from build123d import *

# Parameters (mm, degrees)
SKETCH1_R           = 31.5
BOSS_EXTRUDE1_DEPTH = 55
CUT_EXTRUDE1_START  = 53
SKETCH1_4_R         = 31.5
SKETCH1_4_R_2       = 9
CUT_EXTRUDE1_DEPTH  = 2
SKETCH1_5_R         = 4
BOSS_EXTRUDE2_DEPTH = 29.525
SKETCH1_7_R         = 2
CUT_EXTRUDE2_DEPTH  = 10
CUT_EXTRUDE3_START  = 53
SKETCH1_10_R        = 1.5
CUT_EXTRUDE3_DEPTH  = 5
CHAMFER1_SIZE       = 5
CHAMFER1_SIZE2      = 12
CHAMFER2_SIZE       = 7
CHAMFER2_SIZE2      = 16
BOSS_EXTRUDE4_START = 75
SKETCH1_11_R        = 4
BOSS_EXTRUDE4_DEPTH = 20


with BuildPart() as part:
    # Sketch1 → Boss-Extrude1 (new body)
    with BuildSketch(Plane(origin=(0, 0, 0), x_dir=(1, 0, 0), z_dir=(0, 1, 0))):
        with Locations(Location((0, 0, 0), (0, 0, 270))):
            Circle(SKETCH1_R)
    extrude(amount=BOSS_EXTRUDE1_DEPTH)

    # Sketch1<4> → Cut-Extrude1 (cut)
    with BuildSketch(Plane(origin=(0, 0, 0), x_dir=(1, 0, 0), z_dir=(0, 1, 0)).offset(CUT_EXTRUDE1_START)):
        with Locations(Location((0, 0, 0), (0, 0, 270))):
            Circle(SKETCH1_4_R)
        with Locations(Location((0, 0, 0), (0, 0, 270))):
            Circle(SKETCH1_4_R_2, mode=Mode.SUBTRACT)
    extrude(amount=CUT_EXTRUDE1_DEPTH, mode=Mode.SUBTRACT)

    # Sketch1<5> → Boss-Extrude2 (add)
    with BuildSketch(Plane(origin=(0, 0, 0), x_dir=(1, 0, 0), z_dir=(0, 1, 0))):
        with Locations(Location((0, 0, 0), (0, 0, 270))):
            Circle(SKETCH1_5_R)
    extrude(amount=-BOSS_EXTRUDE2_DEPTH)

    # Sketch1<7> → Cut-Extrude2 (cut)
    with BuildSketch(Plane(origin=(0, 0, 0), x_dir=(1, 0, 0), z_dir=(0, 1, 0))):
        with Locations(Location((22.2, 0, 0), (0, 0, 270))):
            Circle(SKETCH1_7_R)
        with Locations(Location((0, 22.2, 0), (0, 0, 270))):
            Circle(SKETCH1_7_R)
        with Locations(Location((-22.2, 0, 0), (0, 0, 270))):
            Circle(SKETCH1_7_R)
        with Locations(Location((0, -22.2, 0), (0, 0, 270))):
            Circle(SKETCH1_7_R)
    extrude(amount=CUT_EXTRUDE2_DEPTH, mode=Mode.SUBTRACT)

    # Sketch1<10> → Cut-Extrude3 (cut)
    with BuildSketch(Plane(origin=(0, 0, 0), x_dir=(1, 0, 0), z_dir=(0, 1, 0)).offset(CUT_EXTRUDE3_START)):
        with Locations(Location((-11.7, 0, 0), (0, 0, 270))):
            Circle(SKETCH1_10_R)
        with Locations(Location((0, 11.7, 0), (0, 0, 270))):
            Circle(SKETCH1_10_R)
        with BuildLine():
            ThreePointArc((13.2, 0), (11.7, 1.5), (10.2, 0))
            Line((10.2, 0), (13.2, 0))
        make_face()
        with BuildLine():
            Line((13.2, 0), (10.2, 0))
            ThreePointArc((10.2, 0), (11.7, -1.5), (13.2, 0))
        make_face()
        with Locations(Location((0, -11.7, 0), (0, 0, 270))):
            Circle(SKETCH1_10_R)
    extrude(amount=-CUT_EXTRUDE3_DEPTH, mode=Mode.SUBTRACT)

    # Chamfer1
    chamfer1_edges = [part.edges().sort_by_distance(p)[0] for p in [
        (0, 0, -31.5),
    ]]
    chamfer1_side = [part.faces().sort_by_distance(p)[0] for p in [
        (0, 0, -30.609045456),
    ]]
    chamfer(chamfer1_edges, length=CHAMFER1_SIZE, length2=CHAMFER1_SIZE2, reference=chamfer1_side[0])

    # Chamfer2
    chamfer2_edges = [part.edges().sort_by_distance(p)[0] for p in [
        (0, 53, -31.5),
    ]]
    chamfer2_side = [part.faces().sort_by_distance(p)[0] for p in [
        (0, 32.5, -31.5),
    ]]
    chamfer(chamfer2_edges, length=CHAMFER2_SIZE, length2=CHAMFER2_SIZE2, reference=chamfer2_side[0])

    # Sketch1<11> → Boss-Extrude4 (add)
    with BuildSketch(Plane(origin=(0, 0, 0), x_dir=(1, 0, 0), z_dir=(0, 1, 0)).offset(BOSS_EXTRUDE4_START)):
        with Locations(Location((0, 0, 0), (0, 0, 270))):
            Circle(SKETCH1_11_R)
    extrude(amount=-BOSS_EXTRUDE4_DEPTH)


solid = part.part
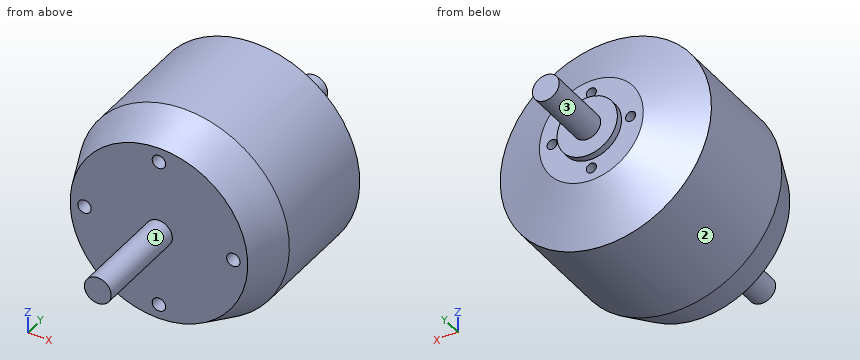
The listing builds one solid part. Answer for the finished solid, in the listing's coordinates (mm). Face numbers are marked on the shaded views. A direction names the side the tool comes from. Round coordinates to 2 decimals unless told otherwise and drop trailing zeros. Write each loop counter-clockwise with the first axis right and the second up, starting at its lowest first coordinate (ties: lowest second). Pieces come first, ordered by that corner, then holes. Notation, with made-up numbers: M 15,36.25 L 56,36.25 A32 cw 56,62.25 Z; hole C 36,-37 d10. An arc over 180 degrees is marked long. Write each question's results on one line, items separated by ' | '. Start each with the question number.
(1) Find the intervals of material crossed by line 1 (Y direction, x = 11.5, z = -6.5); line 2 (X direction, y = 7.25, z = 0); line 3 (X direction, y = 7.5, z = 0) (3 decimals), in increasing order.
(2) The part is cut by section A-A, the plane y = 50.5. Write down the section's boundary in (x, z), and give its area (3 significant figures).
(3) For the marked faces 1, 2 and 3, determine the directions among +Z, -Z, +X, -X, +Y, -Y from which every point of the face is accessible in a straight line to the end or side of a thin tool.
(4) The part is cut by section B-B, the plane y = 29.5. Write down the section's boundary in (x, z), and give its area (3 significant figures).
(5) Each of these flat-tipped pins is pushed along its axis until it touches: P1, Ø5, axis at x = 22.2, z = 0, coming from the +Y side; P2, Ø10, axis at y = 28, z = -24, coming from the +X side; P3, Ø3.5, axis at x = 0, z = -12, coming from the +Y side. Where does it stop, or does it pass through?
Worked answers:
1) line 1: y = 0 to 53 | line 2: x = -29.52 to -24.2, -20.2 to 20.2, 24.2 to 29.52 | line 3: x = -29.625 to -24.2, -20.2 to 20.2, 24.2 to 29.625
2) outline: C 0,0 d42.43; hole C -11.7,0 d3; hole C 0,-11.7 d3; hole C 0,11.7 d3; hole C 11.7,0 d3 | area: 1,390 mm²
3) face 1: -Y | face 2: +Y, -Y | face 3: +Y
4) outline: C 0,0 d63 | area: 3,120 mm²
5) P1: stops at y = 51.16 | P2: stops at x = 25.12 | P3: stops at y = 53
